For this review, use the dimensioned drawing (mm, ordinates from the lowest corner) and the shaded views. Coordinates: 2 decimals unless noted, no trailing zeros. Loops run counter-clockwise (first coordinate to the right, second up) from the corner with the lowest first, then second, coordinate; pieces in that order, holes last.
1. Clearance check with flat-ended pins moving along their axes: P1, Ø3, axis at x = 39.5, y = 3.5, coming from the +Z side; P2, Ø1, axis at y = 3, z = 49.5, coming from the -X side; P3, Ø2, axis at x = 88, y = 1, coming from the +Z side (1 decimal); P4, Ø10, axis at x = 65.33, z = 65.4, coming from the +Y side. State where each tip first meets the part, or that it passes through.
2. To check wall thickness, follow probe 1 along Z at (x, y) = (65.5, 5.5) (1 decimal); probe 2 along Z at (x, y) = (63, 6.25) (1 decimal); probe 3 along Z at (x, y) = (97, 2.75). State the ranges of each line that lie inside material, in increasing order.
3. Take a section at B-B, the plane z = 112.5. State the section outline as (x, y) points.
4. Take a section at C-C, the plane x = 99. State the section outline as (y, z) points.
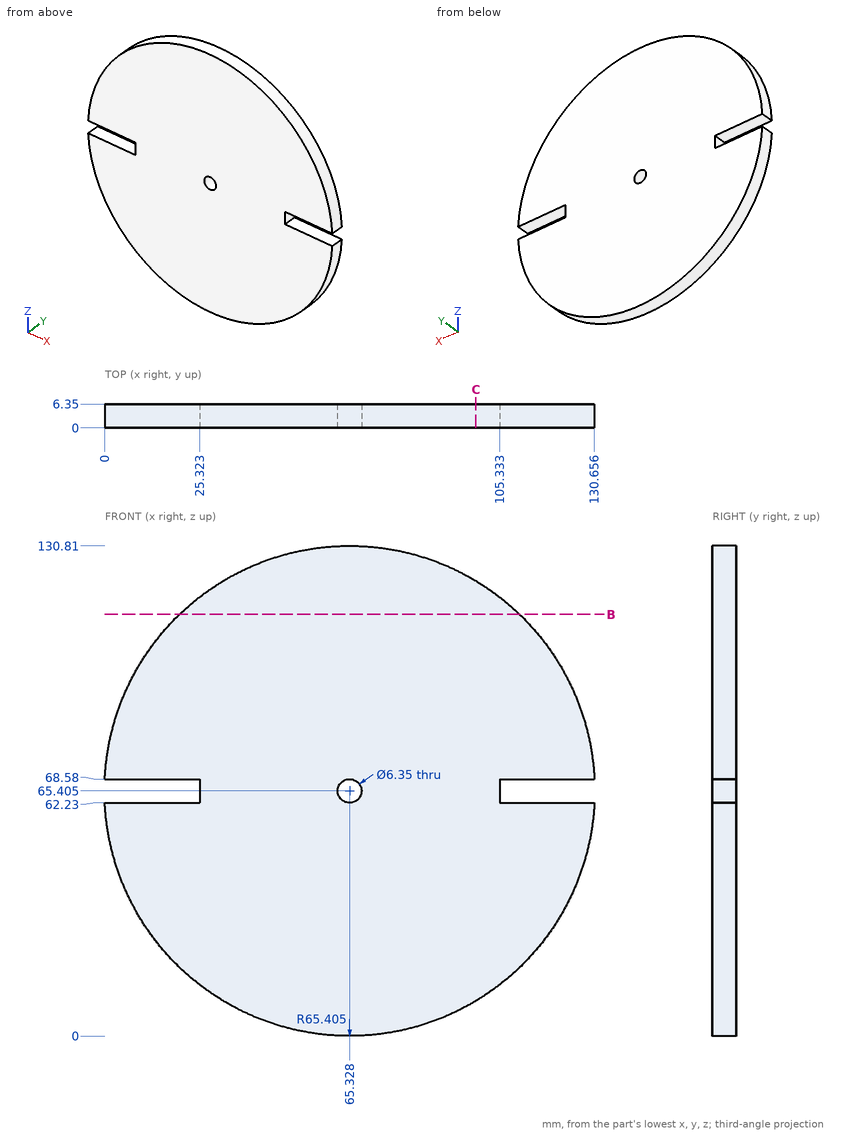
Results list:
1. P1: stops at z = 126.12
1. P2: stops at x = 1.76
1. P3: stops at z = 127.1
1. P4: stops at y = 6.35
2. probe 1: z = 0 to 62.2, 68.6 to 130.8
2. probe 2: z = 0 to 63.2, 67.6 to 130.8
2. probe 3: z = 8.18 to 122.63
3. outline: (19.94, 0) - (110.71, 0) - (110.71, 6.35) - (19.94, 6.35) - close
4. outline: (0, 9.33) - (6.35, 9.33) - (6.35, 121.48) - (0, 121.48) - close
